Input: part model. Units: mm. Frame: model coordinates. Face numbers are marked on the shaded views. A direction names the side the tool comes from. Give positions to 0.01 mm unless a question says otherwise; leave off trailing zeros. Loops run counter-clockwise (first coordinate to the right, second up) from the corner with the lowest first, then second, coordinate; pieces in that order, holes last. Notation, with made-up numbers: M -5,-1 L 48,-1 A17 ccw 48,12 Z; hole C 7.5,80.25 d8. An arc over 180 degrees is marked long. Return JSON: item names as keys, results as strings. Group by question number.
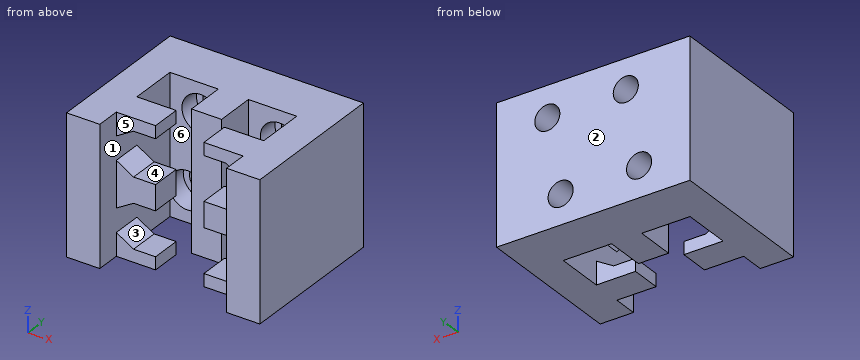
```python
from build123d import *

# Parameters (mm, degrees)
ESQUISSE1_W                   = 30.8
ESQUISSE1_H                   = 24.15
BOSS_EXTRU_1_DEPTH            = 22
ENL_V_START                   = -22
ENL_V_MAT_EXTRU_2_DEPTH       = 22
ENL_V_MAT_EXTRU_14_DEPTH      = 47.950397903
ENL_V_MAT_EXTRU_14_DEPTH_BACK = 4.8
ENL_V_MAT_EXTRU_19_DEPTH      = 4.8
ENL_V_MAT_EXTRU_20_DEPTH      = 4.8
ENL_V_MAT_EXTRU_21_DEPTH      = 4.8
ESQUISSE17_R                  = 2
ENL_V_MAT_EXTRU_22_DEPTH      = 4.4
ESQUISSE18_R                  = 3
ENL_V_MAT_EXTRU_24_DEPTH      = 3.4
ESQUISSE19_R                  = 3
ENL_V_MAT_EXTRU_29_DEPTH      = 3.4
ESQUISSE22_R                  = 3
ENL_V_MAT_EXTRU_30_DEPTH      = 3.4
ESQUISSE23_R                  = 3
ENL_V_MAT_EXTRU_31_DEPTH      = 3.4


# Read off the part's stored shape, not the designer's step: Enlèv. mat.-Extru.2
with BuildPart() as part:
    # Esquisse1 → Boss.-Extru.1 (new body)
    with BuildSketch(Plane.XY):
        with Locations((-20.769736842, 6.111184211)):
            Rectangle(ESQUISSE1_W, ESQUISSE1_H)
    extrude(amount=BOSS_EXTRU_1_DEPTH)

    # Enlèv. mat.-Extru.2 outline → Enlèv. mat.-Extru.2 (cut)
    with BuildSketch(Plane.XY.offset(22).offset(ENL_V_START)):
        Polygon((-30.869736842, -5.963815789), (-10.669736842, -5.963815789), (-10.669736842, -2.113815789), (-16.919736842, -2.113815789), (-16.919736842, 2.686184211), (-10.669736842, 2.686184211), (-10.669736842, 10.386184211), (-18.369736842, 10.386184211), (-18.369736842, 4.136184211), (-23.169736842, 4.136184211), (-23.169736842, 10.386184211), (-30.869736842, 10.386184211), (-30.869736842, 2.686184211), (-24.619736842, 2.686184211), (-24.619736842, -2.113815789), (-30.869736842, -2.113815789), align=None)
    extrude(amount=ENL_V_MAT_EXTRU_2_DEPTH, mode=Mode.SUBTRACT)

    # Esquisse12 → Enlèv. mat.-Extru.14 (cut, two sides: drawn at the far end of the back side and taken through both)
    with BuildSketch(Plane(origin=(0, -2.113815789, 0), x_dir=(-1, 0, 0), z_dir=(0, -1, 0)).offset(-ENL_V_MAT_EXTRU_14_DEPTH_BACK)):
        Polygon((16.919736842, -9), (16.919736842, -2), (13.419736842, -2), (10.669736842, -3.636306817), (10.669736842, -7.363693183), (13.419736842, -9), align=None)
    extrude(amount=ENL_V_MAT_EXTRU_14_DEPTH + ENL_V_MAT_EXTRU_14_DEPTH_BACK, mode=Mode.SUBTRACT)

    # Esquisse13 → Enlèv. mat.-Extru.19 (cut)
    with BuildSketch(Plane(origin=(0, -2.113815789, 0), x_dir=(-1, 0, 0), z_dir=(0, -1, 0))):
        Polygon((24.619736842, -2), (28.119736842, -2), (30.869736842, -3.636306817), (30.869736842, -7.363693183), (28.119736842, -9), (24.619736842, -9), align=None)
    extrude(amount=-ENL_V_MAT_EXTRU_19_DEPTH, mode=Mode.SUBTRACT)

    # Esquisse14 → Enlèv. mat.-Extru.20 (cut)
    with BuildSketch(Plane(origin=(0, -2.113815789, 0), x_dir=(-1, 0, 0), z_dir=(0, -1, 0))):
        Polygon((24.619736842, -20), (28.119736842, -20), (30.869736842, -18.363693183), (30.869736842, -14.636306817), (28.119736842, -13), (24.619736842, -13), align=None)
    extrude(amount=-ENL_V_MAT_EXTRU_20_DEPTH, mode=Mode.SUBTRACT)

    # Esquisse16 → Enlèv. mat.-Extru.21 (cut)
    with BuildSketch(Plane(origin=(0, -2.113815789, 0), x_dir=(-1, 0, 0), z_dir=(0, -1, 0))):
        Polygon((16.919736842, -20), (13.419736842, -20), (10.669736842, -18.363693183), (10.669736842, -14.636306817), (13.419736842, -13), (16.919736842, -13), align=None)
    extrude(amount=-ENL_V_MAT_EXTRU_21_DEPTH, mode=Mode.SUBTRACT)

    # Esquisse17 → Enlèv. mat.-Extru.22 (cut)
    with BuildSketch(Plane(origin=(0, 18.186184211, 0), x_dir=(1, 0, 0), z_dir=(0, 1, 0))):
        with Locations(Location((-15.581044692, -4.75, 0), (0, 0, 270))):
            Circle(ESQUISSE17_R)
        with Locations(Location((-13.462622288, -17.069183679, 0), (0, 0, 270))):
            Circle(ESQUISSE17_R)
        with Locations(Location((-25.961314438, -17.25, 0), (0, 0, 270))):
            Circle(ESQUISSE17_R)
        with Locations(Location((-28.079736842, -4.930816321, 0), (0, 0, 270))):
            Circle(ESQUISSE17_R)
    extrude(amount=-ENL_V_MAT_EXTRU_22_DEPTH, mode=Mode.SUBTRACT)

    # Esquisse18 → Enlèv. mat.-Extru.24 (cut)
    with BuildSketch(Plane(origin=(0, 13.786184211, 0), x_dir=(1, 0, 0), z_dir=(0, 1, 0))):
        with Locations(Location((-28.079736842, -4.930816321, 0), (0, 0, 270))):
            Circle(ESQUISSE18_R)
    extrude(amount=-ENL_V_MAT_EXTRU_24_DEPTH, mode=Mode.SUBTRACT)

    # Esquisse19 → Enlèv. mat.-Extru.29 (cut)
    with BuildSketch(Plane(origin=(0, 13.786184211, 0), x_dir=(1, 0, 0), z_dir=(0, 1, 0))):
        with Locations(Location((-25.961314438, -17.25, 0), (0, 0, 270))):
            Circle(ESQUISSE19_R)
    extrude(amount=-ENL_V_MAT_EXTRU_29_DEPTH, mode=Mode.SUBTRACT)

    # Esquisse22 → Enlèv. mat.-Extru.30 (cut)
    with BuildSketch(Plane(origin=(0, 13.786184211, 0), x_dir=(1, 0, 0), z_dir=(0, 1, 0))):
        with Locations(Location((-15.581044692, -4.75, 0), (0, 0, 270))):
            Circle(ESQUISSE22_R)
    extrude(amount=-ENL_V_MAT_EXTRU_30_DEPTH, mode=Mode.SUBTRACT)

    # Esquisse23 → Enlèv. mat.-Extru.31 (cut)
    with BuildSketch(Plane(origin=(0, 13.786184211, 0), x_dir=(1, 0, 0), z_dir=(0, 1, 0))):
        with Locations(Location((-13.462622288, -17.069183679, 0), (0, 0, 270))):
            Circle(ESQUISSE23_R)
    extrude(amount=-ENL_V_MAT_EXTRU_31_DEPTH, mode=Mode.SUBTRACT)


solid = part.part
```
Item 1: Reachability of the marked faces 4, 5 and 6 from +Z, -Z, +X, -X, +Y, -Y: full face, straight path, thin tool, end or side. Return the list, or none.
Item 2: Section B-B, the plane y = 9. Return loops of the section in (x, z).
Item 3: First-contact query: pin 1 Ø1.8 at (x, z) = (-27, 1) entering from -Y; pin 2 Ø5 at (x, z) = (-28.08, 4.93) entering from -Y. Flat tips, straight axial feed; report the tip coordinate or a pass-through.
Item 4: Section C-C, the plane z = 17.25. Return loops of the section in (x, y).
Item 5: Material intervals for line 1 (X direction, y = 6.25, z = 20.5); line 2 (Z direction, x = -13.5, y = -0.25); line 3 (X direction, y = 12.65, z = 17.25), sorted ascending. Write a range as from..to.
Item 6: Section D-D, the plane z = 20.75. Return loops of the section in (x, y), then the cut area to 3 significant figures.
Item 7: Pull-direction query (Y, two-part tool) for the marked faces 1, 2 and 3; classes: pulls with the +Y half, pulls with the -Y half, needs draft (parallel to the pull), parting line crosses it, or undercut.
Answer below:
{
 "1": {"face 4": "-Y", "face 5": "+Z, -Z, -Y", "face 6": "+Z, -Z"},
 "2": {"outline": "M -36.17,0 L -30.87,0 L -30.87,22 L -36.17,22 Z; M -23.17,0 L -18.37,0 L -18.37,22 L -23.17,22 Z; M -10.67,0 L -5.37,0 L -5.37,22 L -10.67,22 Z"},
 "3": {"pin 1": "y = -2.11", "pin 2": "y = 13.79"},
 "4": {"outline": "M -36.17,-5.96 L -30.87,-5.96 L -30.87,10.39 L -28.96,10.39 L -28.96,13.79 L -27.96,13.79 L -27.96,18.19 L -36.17,18.19 Z; M -23.96,13.79 L -22.96,13.79 L -22.96,10.39 L -23.17,10.39 L -23.17,4.14 L -18.37,4.14 L -18.37,10.39 L -16.46,10.39 L -16.46,13.79 L -15.45,13.79 L -15.45,18.19 L -23.96,18.19 Z; M -11.47,13.79 L -10.47,13.79 L -10.47,10.39 L -10.67,10.39 L -10.67,-5.96 L -5.37,-5.96 L -5.37,18.19 L -11.47,18.19 Z"},
 "5": {"line 1": "-36.17..-30.87, -23.17..-18.37, -10.67..-5.37", "line 2": "0..2, 9..13, 20..22", "line 3": "-36.17..-28.96, -22.96..-16.46, -10.47..-5.37"},
 "6": {"outline": "M -36.17,-5.96 L -30.87,-5.96 L -30.87,-2.11 L -24.62,-2.11 L -24.62,2.69 L -30.87,2.69 L -30.87,10.39 L -23.17,10.39 L -23.17,4.14 L -18.37,4.14 L -18.37,10.39 L -10.67,10.39 L -10.67,2.69 L -16.92,2.69 L -16.92,-2.11 L -10.67,-2.11 L -10.67,-5.96 L -5.37,-5.96 L -5.37,18.19 L -36.17,18.19 Z", "area": "504 mm^2"},
 "7": {"face 1": "undercut", "face 2": "pulls with the +Y half", "face 3": "needs draft"}
}
